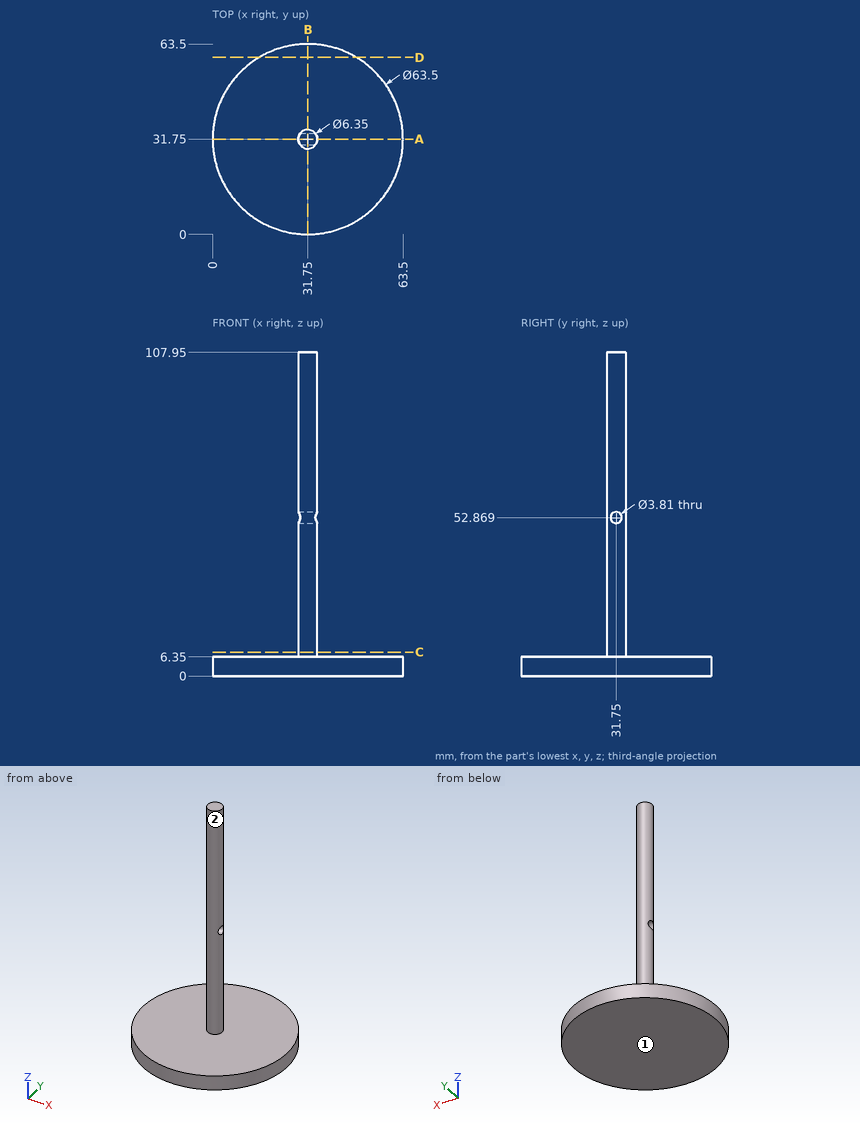
Geometry check sheet. Reference: drawing and pictorial views, mm from the part's lowest x, y, z. A direction names the side the tool comes from. Coordinates: 2 decimals unless noted, no trailing zeros. Order: outer loops, then holes, each group sorted by start corner. A loop starts at its lowest first (then second) coordinate and runs counter-clockwise, first axis right, second up. Notation, with made-up numbers: M 25,43.5 L 63,43.5 A12 cw 63,50.5 Z; hole C 18,72.25 d11. An arc over 180 degrees is marked long. Write each question's results on one line, items separated by ' | '. Start each with the question number.
1. Cross-section at A-A on y = 31.75. Record the cut outline in (x, z) (3 decimals), and give its area (3 significant figures).
2. Cross-section at B-B on x = 31.75. Record the cut outline in (y, z) (3 decimals), and give its area (3 significant figures).
3. Access from +Z, -Z, +X, -X, +Y, -Y to the whole of each face (thin tool, end or side, straight path). Record for the marked faces 1 and 2.
4. Cross-section at C-C on z = 8. Record the cut outline in (x, y) (3 decimals), and give its area (3 significant figures).
5. Cross-section at D-D on y = 59. Record the cut outline in (x, z).
6. Go/stop test with flat-tipped pins: P1, Ø6, axis at x = 13, y = 40.5, coming from the +Z side; P2, Ø8, axis at x = 15, y = 46.5, coming from the -Z side; P3, Ø6, axis at y = 31.75, z = 52.87, coming from the +X side (3 decimals); P4, Ø5, axis at x = 30, z = 53.5, coming from the +Y side (3 decimals). Record where each tip stops, or that it passes through.
7. Material ranges on probe 1 along Z at (x, y) = (33.75, 31.75); probe 2 along Z at (x, y) = (46, 11.5); probe 3 along Y at (x, z) = (34, 95.5), recorded low to high.
Checks:
1) outline: M 0,0 L 63.5,0 L 63.5,6.35 L 34.925,6.35 L 34.925,50.964 L 28.575,50.964 L 28.575,6.35 L 0,6.35 Z; M 28.575,54.774 L 34.925,54.774 L 34.925,107.95 L 28.575,107.95 Z | area: 1,020 mm²
2) outline: M 0,0 L 63.5,0 L 63.5,6.35 L 34.925,6.35 L 34.925,107.95 L 28.575,107.95 L 28.575,6.35 L 0,6.35 Z; hole C 31.75,52.869 d3.81 | area: 1,040 mm²
3) face 1: -Z, +X, -X, +Y, -Y | face 2: +Z
4) outline: C 31.75,31.75 d6.35 | area: 31.7 mm²
5) outline: M 15.46,0 L 48.04,0 L 48.04,6.35 L 15.46,6.35 Z
6) P1: stops at z = 6.35 | P2: stops at z = 0 | P3: stops at x = 34.925 | P4: stops at y = 34.925
7) probe 1: z = 0 to 50.96, 54.77 to 107.95 | probe 2: z = 0 to 6.35 | probe 3: y = 29.51 to 33.99
